Here's how the part is built. I have some questions about the finished solid (model axes, mm). Face numbers are marked on the shaded views. A direction names the side the tool comes from. Give positions to 0.01 mm unless a question says otherwise; leave off trailing zeros. Answer in a Markdown table with one row per item. Add a question column.
Item 1: Which directions (+Z, -Z, +X, -X, +Y, -Y) give clear straight access to the entire face, cutting with the end or side of a thin tool? Please do the marked faces 1, 2 and 3.
Item 2: If I drill on line 1 (Y direction, x = 0, z = 11.25); line 2 (Y direction, x = 4.5, z = 1.5); line 3 (X direction, y = 1.75, z = 1.25), over which ranges is the centre line in solid material (lowest first)?
Item 3: We'd pull the mould along Y, two halves only. Please class the marked faces 4, 5, 6 and 7: released by +Y, released by -Y, zero draft, split by the parting line, or undercut.
Item 4: For P1, Ø6, axis at x = -8, y = 8.5, coming from the -Z side; P2, Ø1, axis at x = 8.5, z = 8, coming from the -Y side; P3, Ø1.5, axis at y = -3.5, z = 9, coming from the -X side, each with a flat end and sliding along its axis, tell me the tip position at first contact or that it passes through.
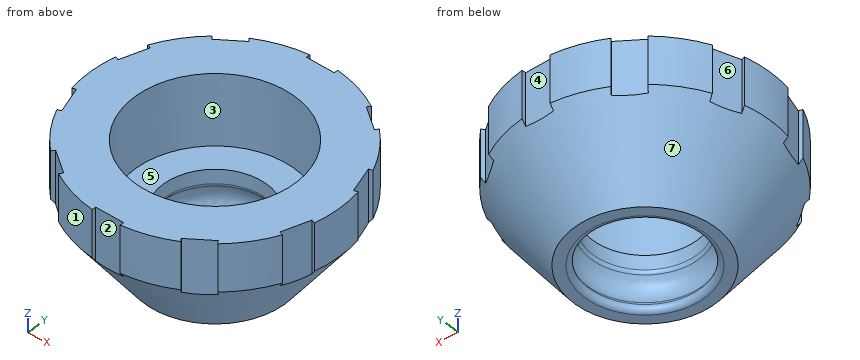
```python
from build123d import *

# Parameters (mm, degrees)
SKETCH005_W        = 3
SKETCH005_H        = 1
POCKET002_DEPTH    = 92.668992
POLARPATTERN_COUNT = 10
FILLET_R           = 0.5
FILLET004_R        = 2


with BuildPart() as part:
    # Sketch003 → Revolution (revolve)
    with BuildSketch(Plane.XZ):
        Polygon((-5.5, 0), (-7.520726, 3.5), (-5.520726, 3.5), (-5.520726, 5.5), (-8.51234, 5.5), (-8.51234, 8), (-8.51234, 13), (-11.31234, 13), (-13.31234, 13), (-13.31234, 8), (-7.5, 0), align=None)
    revolve(axis=Axis((0, 0, 0), (0, 0, 1)))

    # Sketch005 (on Face1 of Revolution) → Pocket002 (cut, through all)
    with BuildSketch(Plane(origin=(0, 0, 13), x_dir=(-1, 0, 0), z_dir=(0, 0, 1))):
        with Locations((0, 13.31234)):
            Rectangle(SKETCH005_W, SKETCH005_H)
    pocket002 = extrude(amount=-POCKET002_DEPTH, mode=Mode.SUBTRACT)

    # PolarPattern: Pocket002 ×10 about axis
    polarpattern_axis = Axis((0, 0, 13), (0, 0, 1))
    for i in range(1, POLARPATTERN_COUNT):
        add(pocket002.rotate(polarpattern_axis, i * 360 / POLARPATTERN_COUNT), mode=Mode.SUBTRACT)

    # Fillet
    fillet_edges = [part.edges().sort_by_distance(p)[0] for p in [
        (5.520726, 0, 3.5),
        (5.5, 0, 0),
    ]]
    fillet(fillet_edges, radius=FILLET_R)

    # Fillet004
    fillet004_edges = [part.edges().sort_by_distance(p)[0] for p in [
        (7.520726, 0, 3.5),
    ]]
    fillet(fillet004_edges, radius=FILLET004_R)


solid = part.part
```
Recorded:
| question | item | result |
|---|---|---|
| 1 | face 1 | +Z, -Z, -X, -Y |
| 1 | face 2 | +Z, -Z, -Y |
| 1 | face 3 | +Z |
| 2 | line 1 | y = -12.81 to -8.51, 8.51 to 12.81 |
| 2 | line 2 | y = -7.32 to -4.42, 4.42 to 7.32 |
| 2 | line 3 | x = -8.22 to -5.96, 5.96 to 8.22 |
| 3 | face 4 | released by +Y |
| 3 | face 5 | undercut |
| 3 | face 6 | undercut |
| 3 | face 7 | split by the parting line |
| 4 | P1 | stops at z = 1.61 |
| 4 | P2 | stops at y = -10.02 |
| 4 | P3 | stops at x = -12.58 |
